```python
from build123d import *

# Parameters (mm, degrees)
CROQUIS1_R              = 0.5
SALIENTE_EXTRUIR1_DEPTH = 1.1
CROQUIS2_W              = 7.5
CROQUIS2_H              = 9
SALIENTE_EXTRUIR2_DEPTH = 3
REDONDEO1_R             = 1.5
CROQUIS3_W              = 6.8
CROQUIS3_H              = 6.8
SALIENTE_EXTRUIR3_DEPTH = 3
REDONDEO2_R             = 0.5
CROQUIS4_W              = 5
CROQUIS4_H              = 3
SALIENTE_EXTRUIR4_DEPTH = 1
SALIENTE_EXTRUIR5_DEPTH = 15
CROQUIS7_R              = 2.1
SALIENTE_EXTRUIR6_DEPTH = 7


with BuildPart() as part:
    # Croquis1 → Saliente-Extruir1 (new body)
    with BuildSketch(Plane(origin=(0, 0, 0), x_dir=(1, 0, 0), z_dir=(0, 1, 0))):
        with BuildLine():
            Line((-12.5, 10), (-1, 10))
            ThreePointArc((-1, 10), (0, 9), (1, 10))
            Line((1, 10), (12.5, 10))
            Line((12.5, 10), (12.5, -10))
            Line((12.5, -10), (1, -10))
            ThreePointArc((1, -10), (0, -9), (-1, -10))
            Line((-1, -10), (-12.5, -10))
            Line((-12.5, -10), (-12.5, 10))
        make_face()
        with Locations(Location((11.5, 2.5, 0), (0, 0, 270))):
            Circle(CROQUIS1_R, mode=Mode.SUBTRACT)
        with Locations(Location((11.5, -2.5, 0), (0, 0, 90))):
            Circle(CROQUIS1_R, mode=Mode.SUBTRACT)
        with Locations(Location((-8.5, 9, 0), (0, 0, 270))):
            Circle(CROQUIS1_R, mode=Mode.SUBTRACT)
        with Locations(Location((-3, 9, 0), (0, 0, 270))):
            Circle(CROQUIS1_R, mode=Mode.SUBTRACT)
    extrude(amount=SALIENTE_EXTRUIR1_DEPTH)


with BuildPart() as body_2:
    # Croquis2 → Saliente-Extruir2 (new body)
    with BuildSketch(Plane(origin=(0, 1.1, 0), x_dir=(1, 0, 0), z_dir=(0, 1, 0))):
        with Locations((-10.25, 0)):
            Rectangle(CROQUIS2_W, CROQUIS2_H)
    extrude(amount=SALIENTE_EXTRUIR2_DEPTH)

    # Redondeo1
    redondeo1_edges = [body_2.edges().sort_by_distance(p)[0] for p in [
        (-10.25, 1.1, -4.5),
        (-10.25, 4.1, -4.5),
        (-10.25, 1.1, 4.5),
        (-10.25, 4.1, 4.5),
    ]]
    fillet(redondeo1_edges, radius=REDONDEO1_R - 0.0001)  # a hair under: the kernel refuses the full size

    # Combinar1: union part
    add(part.part)

    # Croquis3 → Saliente-Extruir3 (add)
    with BuildSketch(Plane(origin=(0, 1.1, 0), x_dir=(1, 0, 0), z_dir=(0, 1, 0))):
        with Locations((5.1, 4.6)):
            Rectangle(CROQUIS3_W, CROQUIS3_H)
    extrude(amount=SALIENTE_EXTRUIR3_DEPTH)

    # Redondeo2
    redondeo2_edges = [body_2.edges().sort_by_distance(p)[0] for p in [
        (8.5, 2.6, -1.2),
        (8.5, 2.6, -8),
        (1.7, 2.6, -8),
        (1.7, 2.6, -1.2),
    ]]
    fillet(redondeo2_edges, radius=REDONDEO2_R)

    # Croquis4 → Saliente-Extruir4 (add)
    with BuildSketch(Plane(origin=(0, 1.1, 0), x_dir=(1, 0, 0), z_dir=(0, 1, 0))):
        with Locations((4.2, -3.5)):
            Rectangle(CROQUIS4_W, CROQUIS4_H)
    extrude(amount=SALIENTE_EXTRUIR4_DEPTH)

    # Croquis6 → Saliente-Extruir5 (add)
    with BuildSketch(Plane.ZY.offset(14)):
        with BuildLine():
            Line((-3, 0.2), (3, 0.2))
            ThreePointArc((3, 0.2), (4.697056275, 0.902943725), (5.4, 2.6))
            ThreePointArc((5.4, 2.6), (4.697056275, 4.297056275), (3, 5))
            Line((3, 5), (-3, 5))
            ThreePointArc((-3, 5), (-4.697056275, 4.297056275), (-5.4, 2.6))
            ThreePointArc((-5.4, 2.6), (-4.697056275, 0.902943725), (-3, 0.2))
        make_face()
    extrude(amount=SALIENTE_EXTRUIR5_DEPTH)

    # Croquis7 → Saliente-Extruir6 (add)
    with BuildSketch(Plane.ZY.offset(29)):
        with Locations((0, 2.6)):
            Circle(CROQUIS7_R)
    extrude(amount=SALIENTE_EXTRUIR6_DEPTH)


solid = body_2.part
```
Geometry check sheet. Reference: the model listing, model coordinates, mm. A direction names the side the tool comes from. Give positions to 0.01 mm unless a question says otherwise; leave off trailing zeros. Write each loop counter-clockwise with the first axis right and the second up, starting at its lowest first coordinate (ties: lowest second). Pieces come first, ordered by that corner, then holes.
1) Release check for a two-part mould opening along Z. For faces 1 (the cylindrical face through (-8.988, 0.542, -9.108)), 2 (the flat face through (6.8, 0.5, 10)), 3 (the cylindrical face through (-2.7, 0.5, -9.4)), 4 (the flat face through (-21, 0.2, 0)) record: pulls with the +Z half, pulls with the -Z half, needs draft (parallel to the pull), parting line crosses it, or undercut.
2) Material ranges on L1, parallel to X at y = 0.45, z = 2.5; L2, parallel to X at y = 3.75, z = -0.25; L3, parallel to X at y = 4.55, z = -0.25, recorded low to high.
3) Section check A-A, the plane x = -3. Record the boundary of the cut face in (y, z).
4) Section check C-C, the plane y = 3.45. Record the boundary of the cut face in (x, z).
5) Section check D-D, the plane z = 0. Record the boundary of the cut face in (x, y).
6) Section check B-B, the plane x = 11.5. Record the boundary of the cut face in (y, z).
7) Gauge pin test, flat ends, axial feed: pin 1 (1.5 mm diameter, centred on y = 3.5, z = -7.5, fed in from -X); pin 2 (2.5 mm diameter, centred on y = 3, z = -1, fed in from +X); pin 3 (10 mm diameter, centred on x = 5.5, z = 3.5, fed in from +Y). Record the tip position at first contact, or that the pin passes through.
8) Access from +Z, -Z, +X, -X, +Y, -Y to the whole of each face (thin tool, end or side, straight path). Record for faces 5 (the flat face through (-6.5, 3, 0)), 6 (the cylindrical face through (-10.2, 3.65, -4.07)), 7 (the flat face through (5, 4.1, -5)), 8 (the cylindrical face through (-10.2, 3.65, 4.07)).
Computed:
1. face 1: undercut
1. face 2: pulls with the +Z half
1. face 3: undercut
1. face 4: needs draft
2. L1: x = -29 to -14, -12.5 to 11, 12 to 12.5
2. L2: x = -36 to -6.5
2. L3: x = -36 to -14
3. outline: (0, -10) - (1.1, -10) - (1.1, -9.5) - (0, -9.5) - close; (0, -8.5) - (1.1, -8.5) - (1.1, 10) - (0, 10) - close
4. outline: (-36, -1.92) - (-29, -1.92) - (-29, -5.24) - (-14, -5.24) - (-14, -4.24) - (-6.5, -4.24) - (-6.5, 4.24) - (-14, 4.24) - (-14, 5.24) - (-29, 5.24) - (-29, 1.92) - (-36, 1.92) - close; (1.7, -7.5) arc R0.5 ccw to (2.2, -8) - (8, -8) arc R0.5 ccw to (8.5, -7.5) - (8.5, -1.7) arc R0.5 ccw to (8, -1.2) - (2.2, -1.2) arc R0.5 ccw to (1.7, -1.7) - close
5. outline: (-36, 0.5) - (-29, 0.5) - (-29, 0.2) - (-14, 0.2) - (-14, 1.1) - (-12.5, 1.1) - (-12.5, 0) - (12.5, 0) - (12.5, 1.1) - (-6.5, 1.1) - (-6.5, 4.1) - (-14, 4.1) - (-14, 5) - (-29, 5) - (-29, 4.7) - (-36, 4.7) - close
6. outline: (0, -10) - (1.1, -10) - (1.1, -3) - (0, -3) - close; (0, -2) - (1.1, -2) - (1.1, 2) - (0, 2) - close; (0, 3) - (1.1, 3) - (1.1, 10) - (0, 10) - close
7. pin 1: stops at x = 1.7
7. pin 2: stops at x = 8.5
7. pin 3: stops at y = 4.1
8. face 5: +Z, -Z, +Y
8. face 6: -Z, +Y
8. face 7: +Z, -Z, +X, +Y
8. face 8: +Z, +X, +Y
